Answer from the drawing. Dimensions are ordinates in mm from the lowest x, y and z of the part. A direction names the side the tool comes from. Give positions to 0.01 mm unless a question says otherwise; leave off trailing zeros. Order: outer loops, then holes, each group sorted by start corner. A loop starts at its lowest first (then second) coordinate and runs counter-clockwise, first axis right, second up.
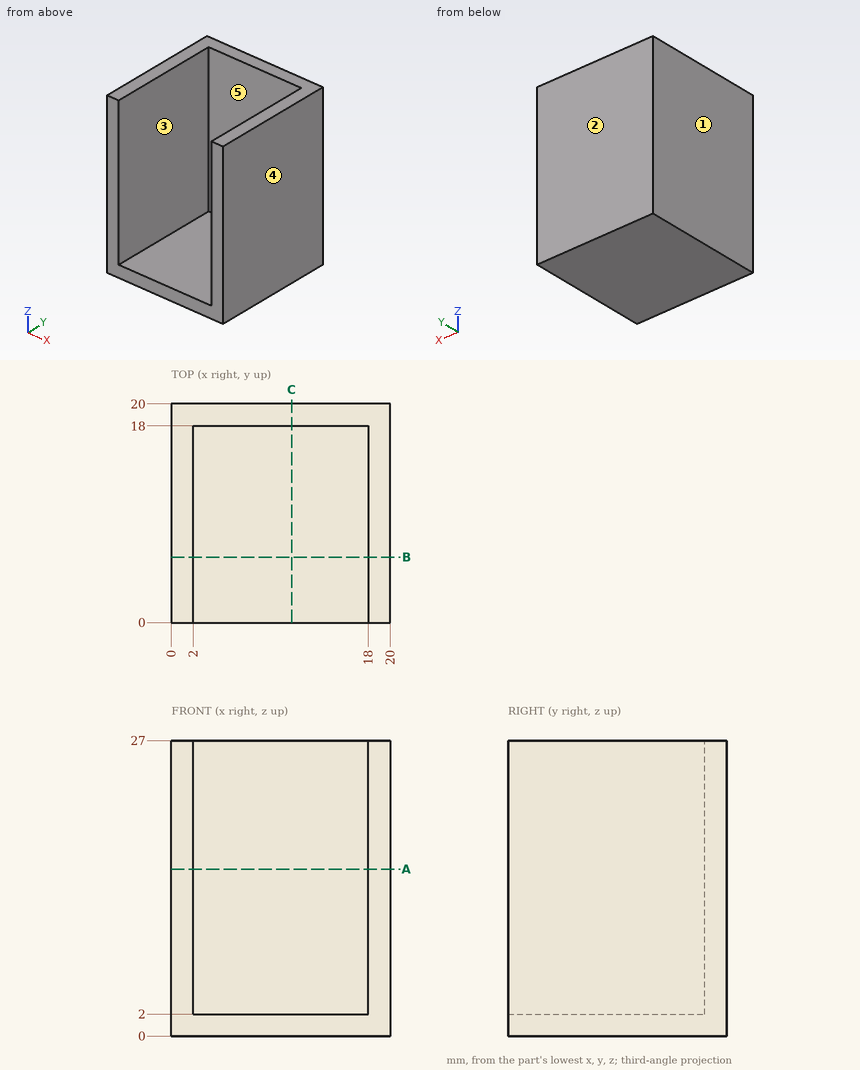
1. The part is cut by section C-C (x = 11). Write down the section's boundary in (y, z), then the cut area to 3 significant figures.
Findings below:
outline: (0, 0) - (20, 0) - (20, 27) - (18, 27) - (18, 2) - (0, 2) - close
area: 90.0 mm2
2. The part is cut by section A-A (z = 15.25). Write down the section's boundary in (x, y), then the cut area to 3 significant figures.
Findings below:
outline: (0, 0) - (2, 0) - (2, 18) - (18, 18) - (18, 0) - (20, 0) - (20, 20) - (0, 20) - close
area: 112 mm2
3. The part is cut by section B-B (y = 6). Write down the section's boundary in (x, z), then the cut area to 3 significant figures.
Findings below:
outline: (0, 0) - (20, 0) - (20, 27) - (18, 27) - (18, 2) - (2, 2) - (2, 27) - (0, 27) - close
area: 140 mm2
4. Given P1, Ø5, axis at x = 11, y = 7.5, coming from the +Z side; P2, Ø3, axis at x = 14.5, z = 16.5, coming from the -Y side, each flat-ended and moving along its own axis, determine where each tip first touches the part or whether it passes through.
Findings below:
P1: stops at z = 2
P2: stops at y = 18
5. Which of the six approach directions +Z, -Z, +X, -X, +Y, -Y give full straight-line access (tool end or side, diameter ignored) to the marked faces 4 and 5?
Findings below:
face 4: +Z, -Z, +X, +Y, -Y
face 5: +Z, -Y
6. The mould has two halves that part along X. Classify the marked faces 1, 2 and 3: pulls with the +X half, pulls with the -X half, needs draft (parallel to the pull), parting line crosses it, or undercut.
Findings below:
face 1: pulls with the -X half
face 2: needs draft
face 3: undercut
7. Straight lines are drawn through the part: probe 1 along X at (y, z) = (12, 4.75); probe 2 along Y at (x, z) = (15, 18.25); probe 3 along Z at (x, y) = (17.5, 17). For each, find the intervals that lie inside material, in ascending order.
Findings below:
probe 1: x = 0 to 2, 18 to 20
probe 2: y = 18 to 20
probe 3: z = 0 to 2
